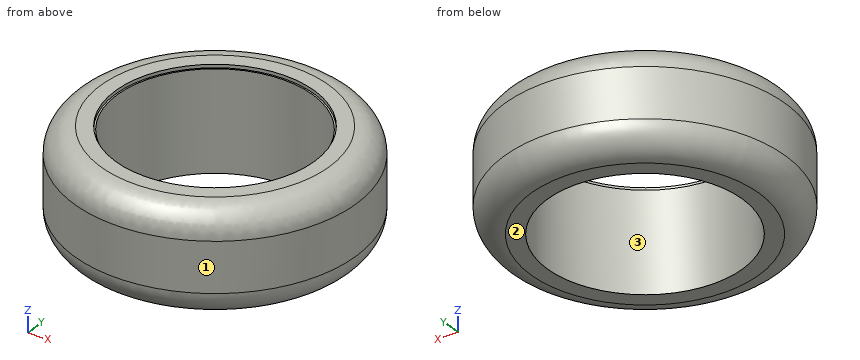
from build123d import *

# Parameters (mm, degrees)
F0_R          = 107.95
F0_R_2        = 74.93
F1_DEPTH      = 76.2
F1_DEPTH_BACK = 2.54
F2_R          = 76.2
F2_R_2        = 74.93
F3_DEPTH      = 2.54
F4_R          = 20.32


with BuildPart() as f1:
    # F0 (on Top) → F1 (new body, two sides)
    with BuildSketch(Plane.XY) as f1_sk:
        Circle(F0_R)
        Circle(F0_R_2, mode=Mode.SUBTRACT)
    extrude(amount=-F1_DEPTH)
    extrude(f1_sk.sketch, amount=F1_DEPTH_BACK)

    # F2 (on face) → F3 (cut)
    with BuildSketch(Plane.XY.offset(2.54)):
        Circle(F2_R)
        Circle(F2_R_2, mode=Mode.SUBTRACT)
    extrude(amount=-F3_DEPTH, mode=Mode.SUBTRACT)

    # F4
    f4_edges = [f1.edges().sort_by_distance(p)[0] for p in [
        (-107.95, 0, 2.54),
        (-107.95, 0, -76.2),
    ]]
    fillet(f4_edges, radius=F4_R)


solid = f1.part
Can you work these out from the model? Positions are in its coordinate system, mm. Face numbers are marked on the shaded views. Coordinates: 2 decimals unless noted, no trailing zeros. Order: outer loops, then holes, each group sorted by start corner. A loop starts at its lowest first (then second) coordinate and runs counter-clockwise, first axis right, second up. Notation, with made-up numbers: M 78,35.5 L 136,35.5 A27 ccw 136,61.5 Z; hole C 64.25,-3 d8. An arc over 180 degrees is marked long. Write item = value, one per line.
(1) If we mould it in two halves opening along Y, with no side actions, what happens to the marked faces 1, 2 and 3? For each: pulls with the +Y half, pulls with the -Y half, needs draft (parallel to the pull), parting line crosses it, or undercut.
Results are:
face_1 = parting line crosses it
face_2 = needs draft
face_3 = undercut
(2) Suppose I cut it at B-B on z = -66. Please give me the cut outline in (x, y).
Results are:
outline = C 0,0 d210.5; hole C 0,0 d149.86
(3) For pin 1 Ø4 at (y, z) = (5.5, -53.5) entering from -X; pin 2 Ø3 at (x, y) = (-63, -81) entering from +Z; pin 3 Ø12 at (y, z) = (26.5, -68) entering from +X, each with a flat end and sliding along its axis, tell me the tip position at first contact or that it passes through.
Results are:
pin_1 = -107.89
pin_2 = -2.58
pin_3 = 104.12
(4) Suppose I cut it at A-A on z = -45. Please give me the cut outline in (x, y).
Results are:
outline = C 0,0 d215.9; hole C 0,0 d149.86
(5) I need wall thicknesses on line 1 along X through (y, z) = (53.5, -53.5); line 2 along Y through (x, z) = (-37.5, -48); line 3 along X through (y, z) = (50, -67). Which ranges of each line are inside material? Lowest first, please. Write a range as [from, to].
Results are:
line_1 = [-93.76, -52.46], [52.46, 93.76]
line_2 = [-101.23, -64.87], [64.87, 101.23]
line_3 = [-91.92, -55.81], [55.81, 91.92]
